Input: part model. Units: mm. Frame: model coordinates. A direction names the side the tool comes from. Give positions to 0.01 mm unless a question says otherwise; leave off trailing zeros. Loops run counter-clockwise (first coordinate to the right, second up) from the corner with the lowest first, then second, coordinate; pieces in that order, holes last.
Solid Edge part; units mm, degrees
sketch "Sketch1" plane through (0, 0, 0) normal (0, 0, 1) x (1, 0, 0)
  line L0 (-7.5, 0) -> (7.5, 0)
  line L1 (7.5, 0) -> (7.5, 19)
  line L2 (7.5, 19) -> (13.5, 19)
  line L3 (13.5, 19) -> (13.5, 29)
  line L4 (13.5, 29) -> (10.5, 29)
  line L5 (10.5, 29) -> (10.5, 22)
  line L6 (10.5, 22) -> (-10.5, 22)
  line L7 (-10.5, 22) -> (-10.5, 29)
  line L8 (-10.5, 29) -> (-13.5, 29)
  line L9 (-13.5, 29) -> (-13.5, 19)
  line L10 (-13.5, 19) -> (-7.5, 19)
  line L11 (-7.5, 19) -> (-7.5, 0)
  dimension "D1" = 7.5
  dimension "D2" = 7.5
  dimension "D3" = 13.5
  dimension "D4" = 13.5
extrude "Protrusion1" add sketch "Sketch1" along normal blind 13
sketch "Sketch2" plane through (0, 0, 0) normal (0, 0, 1) x (1, 0, 0)
  line L0 (-16.5, 21) -> (-16.5, 0)
  line L1 (-16.5, 0) -> (-7.5, 0)
  line L2 (-7.5, 19) -> (-7.5, 0)
  line L3 (-13.5, 19) -> (-7.5, 19)
  line L4 (-13.5, 21) -> (-13.5, 19)
  line L5 (-16.5, 21) -> (-13.5, 21)
  line L6 (7.5, 0) -> (16.5, 0)
  line L7 (16.5, 0) -> (16.5, 21)
  line L8 (16.5, 21) -> (13.5, 21)
  line L9 (13.5, 19) -> (13.5, 21)
  line L10 (7.5, 19) -> (13.5, 19)
  line L11 (7.5, 0) -> (7.5, 19)
extrude "Attachment" add sketch "Sketch2" along normal blind 2
hole "Hole_1" at (13.5, 25, 6.5) direction (-1, 0, 0) diameter 2 end up to next
hole "Hole_2" at (-10.5, 25, 6.5) direction (-1, 0, 0) diameter 1.567 depth 2 thread major 2 thread length 2
hole "Hole___Attachment" at (12, 15, 2) direction (0, 0, -1) diameter 2.6 end up to next
pattern_linear "Pattern1" count 2 spacing 24 along (-1, 0, 0) count 2 spacing 9 along (0, -1, 0) of "Hole___Attachment"
fillet "Round___Attachment" radius 2 4 edges at (16.5, 21, 1) (16.5, 0, 1) (-16.5, 0, 1) (-16.5, 21, 1)
fillet "Round_2" radius 4 4 edges at (-12, 29, 13) (12, 29, 13) (-12, 29, 0) (12, 29, 0)
properties material "ABS Plastic, high impact"
(1) Mould query, pull axis X, two halves, no side actions, for faces 6 (the cylindrical face through (-10.71, 15.17, 1.01)), 7 (the flat face through (-7.5, 10, 7)), 8 (the flat face through (-12, 11, 2)). Classes: +X half, -X half, draft (parallel to the pull), parting line (faces both ways), or undercut.
Values follow:
face 6: undercut
face 7: -X half
face 8: draft
(2) Cut plane D-D (y = 8). Return the cut outline in (x, z), and give its area (3 significant figures).
Values follow:
outline: (-16.5, 0) - (16.5, 0) - (16.5, 2) - (7.5, 2) - (7.5, 13) - (-7.5, 13) - (-7.5, 2) - (-16.5, 2) - close
area: 231 mm2
(3) Cut plane A-A (x = 12). Return the cut outline in (y, z).
Values follow:
outline: (0, 0) - (4.7, 0) - (4.7, 2) - (0, 2) - close; (7.3, 0) - (13.7, 0) - (13.7, 2) - (7.3, 2) - close; (16.3, 0) - (25, 0) arc R4 ccw to (29, 4) - (29, 9) arc R4 ccw to (25, 13) - (19, 13) - (19, 2) - (16.3, 2) - close; hole circle Ø2 at (25, 6.5)
(4) Pin query (flat end, axial travel): pin 1 Ø1.5 at (y, z) = (11.5, 9.5) entering from +X; pin 2 Ø6 at (x, z) = (-2.5, 2.5) entering from +Y; pin 3 Ø1.8 at (x, z) = (-10.5, 5.5) entering from -Y. Return the tip coordinate at first contact, or that it passes through.
Values follow:
pin 1: stops at x = 7.5
pin 2: stops at y = 22
pin 3: stops at y = 19
(5) Cut plane C-C (y = 15). Return the cut outline in (x, z), and give its area (3 significant figures).
Values follow:
outline: (-16.5, 0) - (-13.3, 0) - (-13.3, 2) - (-16.5, 2) - close; (-10.7, 0) - (10.7, 0) - (10.7, 2) - (7.5, 2) - (7.5, 13) - (-7.5, 13) - (-7.5, 2) - (-10.7, 2) - close; (13.3, 0) - (16.5, 0) - (16.5, 2) - (13.3, 2) - close
area: 221 mm2
(6) Reachability of faces 1 (the flat face through (10, 19, 7)), 2 (the flat face through (14, 21, 1)), 3 (the cylindrical face through (12.021, 24.024, 6.717)), 4 (the flat face through (-10.5, 26, 6)), 5 (the flat face through (-11, 19, 7)) from +Z, -Z, +X, -X, +Y, -Y: full face, straight path, thin tool, end or side. Return the list, or none.
Values follow:
face 1: +Z, +X, -Y
face 2: +Z, -Z, +X, +Y
face 3: +X
face 4: +Z, -Z, +Y
face 5: +Z, -X, -Y
(7) Cut plane B-B (z = 6.5). Return the cut outline in (x, y).
Values follow:
outline: (-13.5, 19) - (-7.5, 19) - (-7.5, 0) - (7.5, 0) - (7.5, 19) - (13.5, 19) - (13.5, 24) - (10.5, 24) - (10.5, 22) - (-10.5, 22) - (-10.5, 24.22) - (-12.5, 24.22) - (-12.5, 25.78) - (-10.5, 25.78) - (-10.5, 29) - (-13.5, 29) - close; (10.5, 26) - (13.5, 26) - (13.5, 29) - (10.5, 29) - close
(8) Ray query, probe 1 along X at (y, z) = (15, 1); probe 2 along X at (y, z) = (26.25, 4.25); probe 3 along Z at (x, y) = (-11.8, 25). Return the intervals inside material, ascending.
Values follow:
probe 1: x = -16.5 to -13.3, -10.7 to 10.7, 13.3 to 16.5
probe 2: x = -13.5 to -10.5, 10.5 to 13.5
probe 3: z = 0 to 5.72, 7.28 to 13
